```python
from build123d import *

# Parameters (mm, degrees)
SKETCH1_W           = 6.35
SKETCH1_H           = 76.2
BOSS_EXTRUDE1_DEPTH = 76.2
SKETCH2_W           = 6.35
SKETCH2_H           = 50.8
BOSS_EXTRUDE2_DEPTH = 6.35
SKETCH3_W           = 6.35
SKETCH3_H           = 6.35
SKETCH3_H_2         = 12.7
CUT_EXTRUDE1_DEPTH  = 86.430512699
SKETCH4_W           = 57.15
SKETCH4_H           = 6.35
CUT_EXTRUDE2_DEPTH  = 86.430512699


with BuildPart() as part:
    # Sketch1 → Boss-Extrude1 (new body)
    with BuildSketch(Plane.XY):
        with Locations((9.525, 0)):
            Rectangle(SKETCH1_W, SKETCH1_H)
    extrude(amount=BOSS_EXTRUDE1_DEPTH)

    # Sketch2 → Boss-Extrude2 (add)
    with BuildSketch(Plane.ZY.offset(-6.35)):
        with Locations((-3.175, 0)):
            Rectangle(SKETCH2_W, SKETCH2_H)
    extrude(amount=-BOSS_EXTRUDE2_DEPTH)

    # Sketch3 → Cut-Extrude1 (cut, through all)
    with BuildSketch(Plane.ZY.offset(-6.35)):
        Polygon((69.85, -38.1), (76.2, -38.1), (76.2, -25.4), (69.85, -25.4), (69.85, -31.75), (63.5, -31.75), (63.5, -38.1), align=None)
        with Locations((3.175, -34.925)):
            Rectangle(SKETCH3_W, SKETCH3_H)
        with Locations((73.025, 31.75)):
            Rectangle(SKETCH3_W, SKETCH3_H_2)
    extrude(amount=-CUT_EXTRUDE1_DEPTH, mode=Mode.SUBTRACT)

    # Sketch4 → Cut-Extrude2 (cut, through all)
    with BuildSketch(Plane.ZY.offset(-6.35)):
        with Locations((34.925, 31.75)):
            Rectangle(SKETCH4_W, SKETCH4_H)
    extrude(amount=-CUT_EXTRUDE2_DEPTH, mode=Mode.SUBTRACT)


solid = part.part
```
Geometry: final body of the model. Coordinates: model frame, mm. A direction names the side the tool comes from. Coordinates: 2 decimals unless noted, no trailing zeros. Order: outer loops, then holes, each group sorted by start corner. A loop starts at its lowest first (then second) coordinate and runs counter-clockwise, first axis right, second up. Notation, with made-up numbers: (32.25, 3.25) - (37.25, 3.25) arc R15 cw to (37.25, 19.25) - close; hole circle Ø6 at (8.25, 2). An arc over 180 degrees is marked (long way). Return JSON: item names as keys, results as strings. Group by question number.
1. Cut plane B-B (x = 10.75). Output: boundary loops of the cut face in (y, z) (3 decimals).
2. Cut plane A-A (z = 38.5). Output: boundary loops of the cut face in (x, y) (3 decimals), plus the area to 3 significant figures.
3. Pin query (flat end, axial travel): pin 1 (3 mm diameter, centred on x = 9, z = -3.5, fed in from -Y); pin 2 (1.9 mm diameter, centred on x = 11, y = 34.5, fed in from -Z); pin 3 (1.9 mm diameter, centred on x = 10, z = 3.5, fed in from -Y). Return the tip coordinate at first contact, or that it passes through.
4. Cut plane D-D (z = 68.5). Output: boundary loops of the cut face in (x, y), plus the area to 3 significant figures.
5. Material intervals for line 1 along Y through (x, z) = (11.75, 12) (3 decimals); line 2 along Z through (x, y) = (11.75, 29); line 3 along Y through (x, z) = (11.75, 5), sorted ascending. Write a range as [from, to].
6. Cut plane C-C (y = -33). Output: boundary loops of the cut face in (x, z).
7. Set-up query: faces 1 (the face through (9, -29, 69.85)), 2 (the face through (9, 25.4, -3)), 3 (the face through (9, 25.4, 73)), 4 (the face through (9, 34.925, 35)). Return all of +Z, -Z, +X, -X, +Y, -Y with unobstructed straight access to the full face (end or side cutting, diameter ignored); none if empty.
8. Pull-direction query (Y, two-part tool) for faces 5 (the face through (9, -35, 6.35)), 6 (the face through (9, 32, 6.35)), 7 (the face through (9, -25.4, 73)); classes: pulls with the +Y half, pulls with the -Y half, needs draft (parallel to the pull), parting line crosses it, or undercut.
Resolved:
{
 "1": {"outline": "(-38.1, 6.35) - (-31.75, 6.35) - (-31.75, 0) - (-25.4, 0) - (-25.4, -6.35) - (25.4, -6.35) - (25.4, 0) - (38.1, 0) - (38.1, 69.85) - (25.4, 69.85) - (25.4, 76.2) - (-25.4, 76.2) - (-25.4, 69.85) - (-31.75, 69.85) - (-31.75, 63.5) - (-38.1, 63.5) - close; hole (28.575, 6.35) - (34.925, 6.35) - (34.925, 63.5) - (28.575, 63.5) - close"},
 "2": {"outline": "(6.35, -38.1) - (12.7, -38.1) - (12.7, 28.575) - (6.35, 28.575) - close; (6.35, 34.925) - (12.7, 34.925) - (12.7, 38.1) - (6.35, 38.1) - close", "area": "444 mm²"},
 "3": {"pin 1": "stops at y = -25.4", "pin 2": "stops at z = 0", "pin 3": "stops at y = -31.75"},
 "4": {"outline": "(6.35, -31.75) - (12.7, -31.75) - (12.7, 38.1) - (6.35, 38.1) - close", "area": "444 mm²"},
 "5": {"line 1": "y = [-38.1, 28.575], [34.925, 38.1]", "line 2": "z = [0, 6.35], [63.5, 69.85]", "line 3": "y = [-31.75, 38.1]"},
 "6": {"outline": "(6.35, 6.35) - (12.7, 6.35) - (12.7, 63.5) - (6.35, 63.5) - close"},
 "7": {"face 1": "+Z, +X, -X, -Y", "face 2": "-Z, +X, -X, +Y", "face 3": "+Z, +X, -X, +Y", "face 4": "+X, -X"},
 "8": {"face 5": "needs draft", "face 6": "undercut", "face 7": "pulls with the -Y half"}
}
